from build123d import *

# Parameters (mm, degrees)
SKETCH1_W           = 42
SKETCH1_H           = 42
NEMA_17_DEPTH       = 8
CHAMFER1_SIZE       = 5.5
SKETCH2_R           = 1.5
M3_BOLT_HOLES_DEPTH = 31.757112998
SKETCH3_R           = 16
CUT_EXTRUDE1_DEPTH  = 0.2
SKETCH4_R           = 11.25
BOSS_EXTRUDE1_DEPTH = 0.8
SKETCH5_R           = 11
BOSS_EXTRUDE2_DEPTH = 2
SKETCH6_R           = 3.5
CUT_EXTRUDE2_DEPTH  = 31.918602814
SKETCH7_R           = 2.5
BOSS_EXTRUDE3_DEPTH = 24
CUT_EXTRUDE3_START  = -20
CUT_EXTRUDE3_DEPTH  = 20
SKETCH10_R          = 1.5
BOSS_EXTRUDE4_DEPTH = 1


with BuildPart() as part:
    # Sketch1 → Nema 17 (new body)
    with BuildSketch(Plane(origin=(0, 0, 0), x_dir=(1, 0, 0), z_dir=(0, 1, 0))):
        Rectangle(SKETCH1_W, SKETCH1_H)
    extrude(amount=NEMA_17_DEPTH)

    # Chamfer1
    chamfer1_edges = [part.edges().sort_by_distance(p)[0] for p in [
        (21, 4, 21),
        (-21, 4, 21),
        (-21, 4, -21),
        (21, 4, -21),
    ]]
    chamfer(chamfer1_edges, length=CHAMFER1_SIZE)

    # Sketch2 → M3 Bolt Holes (cut, through all)
    with BuildSketch(Plane.XZ):
        with Locations(Location((-15.5, -15.5, 0), (0, 0, 270))):
            Circle(SKETCH2_R)
        with Locations(Location((15.5, -15.5, 0), (0, 0, 90))):
            Circle(SKETCH2_R)
        with Locations(Location((-15.5, 15.5, 0), (0, 0, 90))):
            Circle(SKETCH2_R)
        with Locations(Location((15.5, 15.5, 0), (0, 0, 270))):
            Circle(SKETCH2_R)
    extrude(amount=-M3_BOLT_HOLES_DEPTH, mode=Mode.SUBTRACT)

    # Sketch3 → Cut-Extrude1 (cut)
    with BuildSketch(Plane(origin=(0, 8, 0), x_dir=(1, 0, 0), z_dir=(0, 1, 0))):
        with Locations(Location((0, 0, 0), (0, 0, 270))):
            Circle(SKETCH3_R)
    extrude(amount=-CUT_EXTRUDE1_DEPTH, mode=Mode.SUBTRACT)

    # Sketch4 → Boss-Extrude1 (add)
    with BuildSketch(Plane(origin=(0, 7.8, 0), x_dir=(1, 0, 0), z_dir=(0, 1, 0))):
        with Locations(Location((0, 0, 0), (0, 0, 270))):
            Circle(SKETCH4_R)
    extrude(amount=BOSS_EXTRUDE1_DEPTH)

    # Sketch5 → Boss-Extrude2 (add)
    with BuildSketch(Plane(origin=(0, 8.6, 0), x_dir=(1, 0, 0), z_dir=(0, 1, 0))):
        with Locations(Location((0, 0, 0), (0, 0, 270))):
            Circle(SKETCH5_R)
    extrude(amount=BOSS_EXTRUDE2_DEPTH)

    # Sketch6 → Cut-Extrude2 (cut, through all)
    with BuildSketch(Plane(origin=(0, 8.6, 0), x_dir=(1, 0, 0), z_dir=(0, 1, 0))):
        with Locations(Location((0, 0, 0), (0, 0, 270))):
            Circle(SKETCH6_R)
    extrude(amount=CUT_EXTRUDE2_DEPTH, mode=Mode.SUBTRACT)

    # Sketch7 → Boss-Extrude3 (add)
    with BuildSketch(Plane(origin=(0, 8.6, 0), x_dir=(1, 0, 0), z_dir=(0, 1, 0))):
        with Locations(Location((0, 0, 0), (0, 0, 270))):
            Circle(SKETCH7_R)
    extrude(amount=BOSS_EXTRUDE3_DEPTH)

    # Sketch9 → Cut-Extrude3 (cut)
    with BuildSketch(Plane(origin=(0, 32.6, 0), x_dir=(1, 0, 0), z_dir=(0, 1, 0)).offset(CUT_EXTRUDE3_START)):
        with BuildLine():
            Line((2, 1.5), (2, -1.5))
            ThreePointArc((2, -1.5), (2.5, 0), (2, 1.5))
        make_face()
    extrude(amount=CUT_EXTRUDE3_DEPTH, mode=Mode.SUBTRACT)

    # Sketch10 → Boss-Extrude4 (add)
    with BuildSketch(Plane.XZ):
        with Locations(Location((15.5, 15.5, 0), (0, 0, 270))):
            Circle(SKETCH10_R)
        with Locations(Location((-15.5, -15.5, 0), (0, 0, 270))):
            Circle(SKETCH10_R)
        with Locations(Location((15.5, -15.5, 0), (0, 0, 270))):
            Circle(SKETCH10_R)
        with Locations(Location((-15.5, 15.5, 0), (0, 0, 270))):
            Circle(SKETCH10_R)
    extrude(amount=-BOSS_EXTRUDE4_DEPTH)


solid = part.part
CAD build for the part. Positions are in the model's coordinates, mm. A direction names the side the tool comes from. Give positions to 0.01 mm unless a question says otherwise; leave off trailing zeros. Loops run counter-clockwise (first coordinate to the right, second up) from the corner with the lowest first, then second, coordinate; pieces in that order, holes last. Notation, with made-up numbers: M 36.5,-12 L 57.5,-12 A16 ccw 57.5,11 Z; hole C 61,53.25 d6. An arc over 180 degrees is marked long. Answer in a Markdown table with one row per item. Add a question column.
Item 1: Band-saw the part on B-B on z = 0. Give the cut face in (x, y).
Item 2: Band-saw the part on D-D on y = 22. Give the cut face in (x, z), then the cut area to 3 significant figures.
Item 3: Tool access for faces 1 (the face through (-15.43, 4.45, -14)), 2 (the face through (0, 32.6, 0)): list every direction of +Z, -Z, +X, -X, +Y, -Y with a clear straight run to the whole face (end or side of a thin tool).
Item 4: Band-saw the part on A-A on y = 7. Give the cut face in (x, z), then the cut area to 3 significant figures.
Item 5: Mould opens along X. For faces 3 (the face through (16, 1, 16)), 4 (the face through (-10.74, 9.59, -2.38)), 5 (the face through (21, 4, 0)) say: +X half, -X half, draft (parallel to the pull), parting line (faces both ways), or undercut.
Item 6: Probe probe 1 along X at (y, z) = (6.75, 15.5); probe 2 along Y at (x, z) = (11, -13); probe 3 along X at (y, z) = (25.5, -2). List the from-to ranges inside material, lowest first.
Item 7: Band-saw the part on C-C on x = 0. Give the cut face in (y, z).
Item 8: Drop flat-ended pins along their axis: P1, Ø4, axis at x = -6, z = 1.5, coming from the -Y side; P2, Ø1.8, axis at x = 15.5, z = -15.5, coming from the +Y side; P3, Ø2, axis at x = -4.5, z = 6.5, coming from the +Y side; P4, Ø3.5, axis at x = 16, z = -15.5, coming from the +Y side. Give the stop position or say it passes through.
Reply:
| question | item | result |
|---|---|---|
| 1 | outline | M -21,0 L 21,0 L 21,8 L 16,8 L 16,7.8 L 11.25,7.8 L 11.25,8.6 L 11,8.6 L 11,10.6 L 3.5,10.6 L 3.5,8.6 L 2.5,8.6 L 2.5,12.6 L 2,12.6 L 2,32.6 L -2.5,32.6 L -2.5,8.6 L -3.5,8.6 L -3.5,10.6 L -11,10.6 L -11,8.6 L -11.25,8.6 L -11.25,7.8 L -16,7.8 L -16,8 L -21,8 Z |
| 2 | outline | M 2,-1.5 L 2,1.5 A2.5 ccw long Z |
| 2 | area | 18.6 mm^2 |
| 3 | face 1 | +Y |
| 3 | face 2 | +Z, -Z, +X, -X, +Y |
| 4 | outline | M -21,-15.5 L -15.5,-21 L 15.5,-21 L 21,-15.5 L 21,15.5 L 15.5,21 L -15.5,21 L -21,15.5 Z; hole C -15.5,-15.5 d3; hole C -15.5,15.5 d3; hole C 15.5,-15.5 d3; hole C 15.5,15.5 d3 |
| 4 | area | 1,680 mm^2 |
| 5 | face 3 | undercut |
| 5 | face 4 | parting line |
| 5 | face 5 | +X half |
| 6 | probe 1 | x = -21 to -17, -14 to 14, 17 to 21 |
| 6 | probe 2 | y = 0 to 8 |
| 6 | probe 3 | x = -1.5 to 1.5 |
| 7 | outline | M 0,-21 L 8,-21 L 8,-16 L 7.8,-16 L 7.8,-11.25 L 8.6,-11.25 L 8.6,-11 L 10.6,-11 L 10.6,-3.5 L 8.6,-3.5 L 8.6,-2.5 L 32.6,-2.5 L 32.6,2.5 L 8.6,2.5 L 8.6,3.5 L 10.6,3.5 L 10.6,11 L 8.6,11 L 8.6,11.25 L 7.8,11.25 L 7.8,16 L 8,16 L 8,21 L 0,21 Z |
| 8 | P1 | stops at y = 0 |
| 8 | P2 | stops at y = 1 |
| 8 | P3 | stops at y = 10.6 |
| 8 | P4 | stops at y = 8 |
